```python
from build123d import *

# Parameters (mm, degrees)
SKETCH_1_W               = 114
SKETCH_1_H               = 95
EXTRUDE_1_DEPTH          = 60
SKETCH_7_W               = 114
SKETCH_7_H               = 25
EXTRUDE_3_DEPTH          = 10
SKETCH_14_R              = 7.5
CUT_EXTRUDE_9_DEPTH      = 50
SKETCH_15_R              = 3.3
CUT_EXTRUDE_10_DEPTH     = 50
MIRROR_2_COPY_1_SKETCH_R = 7.5
MIRROR_2_COPY_1_DEPTH    = 50
MIRROR_2_COPY_2_SKETCH_R = 3.3
MIRROR_2_COPY_2_DEPTH    = 50
CUT_EXTRUDE_8_DEPTH      = 10
SKETCH_16_R              = 3
CUT_EXTRUDE_11_DEPTH     = 50


with BuildPart() as part:
    # 草图1 → 凸台-拉伸1 (new body)
    with BuildSketch(Plane(origin=(0, 0, 0), x_dir=(1, 0, 0), z_dir=(0, 1, 0))):
        Rectangle(SKETCH_1_W, SKETCH_1_H)
    extrude(amount=EXTRUDE_1_DEPTH)

    # 草图7 → 凸台-拉伸3 (add)
    with BuildSketch(Plane(origin=(0, 60, 0), x_dir=(1, 0, 0), z_dir=(0, 1, 0))):
        with Locations((0, -60)):
            Rectangle(SKETCH_7_W, SKETCH_7_H)
        Polygon((-82, -72.5), (-82, 47.5), (-57, 47.5), (-57, -47.5), (-57, -72.5), align=None)
        Polygon((57, -72.5), (82, -72.5), (82, 47.5), (57, 47.5), (57, -47.5), align=None)
    extrude(amount=-EXTRUDE_3_DEPTH)

    # 草图14 → 切除-拉伸9 (cut)
    with BuildSketch(Plane(origin=(0, 60, 0), x_dir=(1, 0, 0), z_dir=(0, 1, 0))):
        with Locations(Location((-40, -37.5, 0), (0, 0, 270))):
            Circle(SKETCH_14_R)
    cut_extrude_9 = extrude(amount=-CUT_EXTRUDE_9_DEPTH, mode=Mode.SUBTRACT)

    # 草图15 → 切除-拉伸10 (cut)
    with BuildSketch(Plane(origin=(0, 10, 0), x_dir=(1, 0, 0), z_dir=(0, 1, 0))):
        with Locations(Location((-40, -37.5, 0), (0, 0, 270))):
            Circle(SKETCH_15_R)
    cut_extrude_10 = extrude(amount=-CUT_EXTRUDE_10_DEPTH, mode=Mode.SUBTRACT)

    # 镜向1: 切除-拉伸9, 切除-拉伸10 across plane
    add(cut_extrude_9.mirror(Plane(origin=(0, 0, 0), x_dir=(0, 0, 1), z_dir=(1, 0, 0))), mode=Mode.SUBTRACT)
    add(cut_extrude_10.mirror(Plane(origin=(0, 0, 0), x_dir=(0, 0, 1), z_dir=(1, 0, 0))), mode=Mode.SUBTRACT)

    # 镜向2: 切除-拉伸9, 切除-拉伸10 across plane
    add(cut_extrude_9.mirror(Plane.XY), mode=Mode.SUBTRACT)
    add(cut_extrude_10.mirror(Plane.XY), mode=Mode.SUBTRACT)

    # 镜向2 copy 1 sketch → 镜向2 copy 1 (cut)
    with BuildSketch(Plane(origin=(0, 60, 0), x_dir=(-1, 0, 0), z_dir=(0, 1, 0))):
        with Locations(Location((-40, -37.5, 0), (0, 0, 270))):
            Circle(MIRROR_2_COPY_1_SKETCH_R)
    extrude(amount=-MIRROR_2_COPY_1_DEPTH, mode=Mode.SUBTRACT)

    # 镜向2 copy 2 sketch → 镜向2 copy 2 (cut)
    with BuildSketch(Plane(origin=(0, 10, 0), x_dir=(-1, 0, 0), z_dir=(0, 1, 0))):
        with Locations(Location((-40, -37.5, 0), (0, 0, 270))):
            Circle(MIRROR_2_COPY_2_SKETCH_R)
    extrude(amount=-MIRROR_2_COPY_2_DEPTH, mode=Mode.SUBTRACT)

    # 草图13 → 切除-拉伸8 (cut)
    with BuildSketch(Plane.XZ.offset(-50)):
        with BuildLine():
            Line((-42, 59.25), (42, 59.25))
            ThreePointArc((42, 59.25), (45.25, 62.5), (42, 65.75))
            Line((42, 65.75), (-42, 65.75))
            ThreePointArc((-42, 65.75), (-45.25, 62.5), (-42, 59.25))
        make_face()
    extrude(amount=-CUT_EXTRUDE_8_DEPTH, mode=Mode.SUBTRACT)

    # 草图16 → 切除-拉伸11 (cut)
    with BuildSketch(Plane.XZ.offset(-50)):
        with Locations(Location((-72, -17.5, 0), (0, 0, 270))):
            Circle(SKETCH_16_R)
        with Locations(Location((-72, 42.5, 0), (0, 0, 270))):
            Circle(SKETCH_16_R)
    cut_extrude_11 = extrude(amount=-CUT_EXTRUDE_11_DEPTH, mode=Mode.SUBTRACT)

    # 镜向3: 切除-拉伸11 across plane
    add(cut_extrude_11.mirror(Plane(origin=(0, 0, 0), x_dir=(0, 0, 1), z_dir=(1, 0, 0))), mode=Mode.SUBTRACT)


solid = part.part
```
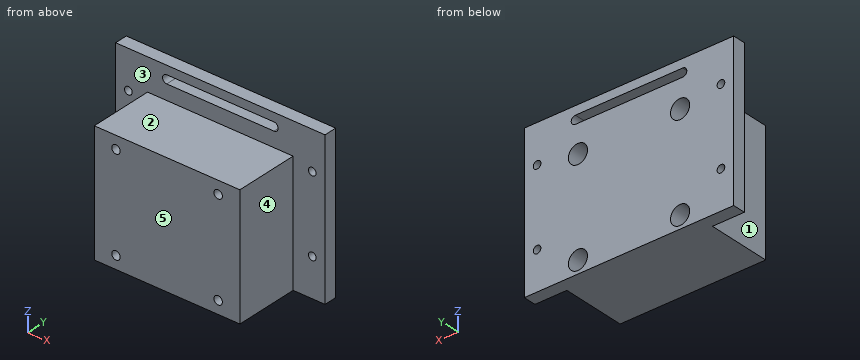
Geometry check sheet. Reference: the model listing, model coordinates, mm. Face numbers are marked on the shaded views. A direction names the side the tool comes from. Give positions to 0.01 mm unless a question says otherwise; leave off trailing zeros. Write each loop counter-clockwise with the first axis right and the second up, starting at its lowest first coordinate (ties: lowest second). Pieces come first, ordered by that corner, then holes. Notation, with made-up numbers: (21.25, 6) - (38.25, 6) arc R32 cw to (38.25, 40) - close; hole circle Ø1 at (18.5, 17.25). An arc over 180 degrees is marked (long way). Use a Markdown table: item, result.
Q1. Set-up check for the marked faces 1, 2, 3, 4 and 5: record each of +Z, -Z, +X, -X, +Y, -Y from which the full face is reachable in a straight line by a thin tool's end or side.
Computed:
| item | result |
|---|---|
| face 1 | +Z, -Z, -X, -Y |
| face 2 | +Z, +X, -X, -Y |
| face 3 | +Z, -Y |
| face 4 | +Z, -Z, +X, -Y |
| face 5 | +Z, -Z, +X, -X, -Y |
Q2. Go/stop test with flat-tipped pins: P1, Ø4.5, axis at x = -43, z = -40, coming from the +Y side; P2, Ø1, axis at y = 12, z = -5, coming from the -X side; P3, Ø15, axis at y = 28, z = -4.5, coming from the +X side. Record where each tip stops, or that it passes through.
Computed:
| item | result |
|---|---|
| P1 | stops at y = 10 |
| P2 | stops at x = -57 |
| P3 | stops at x = 57 |
Q3. Thickness scan on L1, parallel to Z at x = 40, y = 41.5; L2, parallel to X at y = 7, z = -37; L3, parallel to Z at x = 72, y = 54. Record the ranges inside material, lowest first. Write a range as [from, to].
Computed:
| item | result |
|---|---|
| L1 | z = [-47.5, -45], [-30, 30], [45, 47.5] |
| L2 | x = [-57, -43.26], [-36.74, 36.74], [43.26, 57] |
| L3 | z = [-47.5, -20.5], [-14.5, 39.5], [45.5, 72.5] |
Q4. Section check B-B, the plane y = 5. Enter the section's corners in (x, z).
Computed:
| item | result |
|---|---|
| outline | (-57, -47.5) - (57, -47.5) - (57, 47.5) - (-57, 47.5) - close; hole circle Ø6.6 at (-40, -37.5); hole circle Ø6.6 at (-40, 37.5); hole circle Ø6.6 at (40, -37.5); hole circle Ø6.6 at (40, 37.5) |
Q5. Section check C-C, the plane x = 24.5. Enter the section's corners in (y, z).
Computed:
| item | result |
|---|---|
| outline | (0, -47.5) - (60, -47.5) - (60, 59.25) - (50, 59.25) - (50, 47.5) - (0, 47.5) - close; (50, 65.75) - (60, 65.75) - (60, 72.5) - (50, 72.5) - close |
Q6. Section check A-A, the plane z = 62.5. Enter the section's corners in (x, y).
Computed:
| item | result |
|---|---|
| outline | (-82, 50) - (-45.25, 50) - (-45.25, 60) - (-82, 60) - close; (45.25, 50) - (82, 50) - (82, 60) - (45.25, 60) - close |
Q7. Section check D-D, the plane x = -40. Enter the section's corners in (y, z), then the cut area to 3 significant figures.
Computed:
| item | result |
|---|---|
| outline | (0, -47.5) - (60, -47.5) - (60, -45) - (10, -45) - (10, -40.8) - (0, -40.8) - close; (0, -34.2) - (10, -34.2) - (10, -30) - (60, -30) - (60, 30) - (10, 30) - (10, 34.2) - (0, 34.2) - close; (0, 40.8) - (10, 40.8) - (10, 45) - (60, 45) - (60, 59.25) - (50, 59.25) - (50, 47.5) - (0, 47.5) - close; (50, 65.75) - (60, 65.75) - (60, 72.5) - (50, 72.5) - close |
| area | 4,250 mm² |
